```python
from build123d import *

# Parameters (mm, degrees)
SKETCH1_W                = 14
SKETCH1_H                = 99
BOSS_EXTRUDE1_DEPTH      = 40
CUT_EXTRUDE1_DEPTH       = 108.689368092
SKETCH3_W                = 6
SKETCH3_H                = 5
BOSS_EXTRUDE2_DEPTH      = 6
SKETCH4_R                = 1
CUT_EXTRUDE2_DEPTH       = 6
SKETCH5_R                = 1
CUT_EXTRUDE3_DEPTH       = 6
FILLET1_R                = 2
SKETCH6_W                = 6
SKETCH6_H                = 5
BOSS_EXTRUDE3_DEPTH      = 6
SKETCH7_R                = 1
CUT_EXTRUDE4_DEPTH       = 5
SKETCH8_R                = 1
CUT_EXTRUDE5_DEPTH       = 5
FILLET2_R                = 2
SKETCH9_W                = 11
SKETCH9_H                = 5.6
CUT_EXTRUDE6_DEPTH       = 10
BOSS_EXTRUDE4_DEPTH      = 4
BOSS_EXTRUDE4_DEPTH_BACK = 7
FILLET4_R                = 4
SKETCH11_W               = 14.2
SKETCH11_H               = 1.6
BOSS_EXTRUDE5_DEPTH      = 5
SKETCH12_W               = 2
SKETCH12_H               = 2.5
BOSS_EXTRUDE6_DEPTH      = 1
SKETCH13_W               = 2
SKETCH13_H               = 2.5
BOSS_EXTRUDE7_DEPTH      = 1
BOSS_EXTRUDE8_DEPTH      = 10
BOSS_EXTRUDE9_DEPTH      = 10


with BuildPart() as part:
    # Sketch1 → Boss-Extrude1 (new body)
    with BuildSketch(Plane(origin=(0, 0, 0), x_dir=(1, 0, 0), z_dir=(0, 1, 0))):
        with Locations((7, 49.5)):
            Rectangle(SKETCH1_W, SKETCH1_H)
    extrude(amount=BOSS_EXTRUDE1_DEPTH)

    # Sketch2 → Cut-Extrude1 (cut, through all)
    with BuildSketch(Plane.XY):
        with BuildLine():
            Line((14, 0), (14, 40))
            Line((14, 40), (2, 40))
            add(Edge.make_bspline(
                [(2, 40), (2.539521764, 17.05373231), (14, 0)],
                knots=[0, 0, 0, 0.735735095, 0.735735095, 0.735735095], degree=2))
        make_face()
    extrude(amount=-CUT_EXTRUDE1_DEPTH, mode=Mode.SUBTRACT)

    # Sketch3 → Boss-Extrude2 (add)
    with BuildSketch(Plane.ZY):
        with Locations((-84.5, 10)):
            Rectangle(SKETCH3_W, SKETCH3_H)
        with Locations((-14.5, 10)):
            Rectangle(SKETCH3_W, SKETCH3_H)
    extrude(amount=BOSS_EXTRUDE2_DEPTH)

    # Sketch4 → Cut-Extrude2 (cut)
    with BuildSketch(Plane.XZ.offset(-7.5)):
        with Locations(Location((-3, -84.5, 0), (0, 0, 270))):
            Circle(SKETCH4_R)
    extrude(amount=-CUT_EXTRUDE2_DEPTH, mode=Mode.SUBTRACT)

    # Sketch5 → Cut-Extrude3 (cut)
    with BuildSketch(Plane.XZ.offset(-7.5)):
        with Locations(Location((-3, -14.5, 0), (0, 0, 270))):
            Circle(SKETCH5_R)
    extrude(amount=-CUT_EXTRUDE3_DEPTH, mode=Mode.SUBTRACT)

    # Fillet1
    fillet1_edges = [part.edges().sort_by_distance(p)[0] for p in [
        (0, 10, -81.5),
        (0, 10, -87.5),
        (-6, 10, -81.5),
        (-6, 10, -87.5),
        (0, 10, -17.5),
        (0, 10, -11.5),
        (-6, 10, -17.5),
        (-6, 10, -11.5),
    ]]
    fillet(fillet1_edges, radius=FILLET1_R)

    # Sketch6 → Boss-Extrude3 (add)
    with BuildSketch(Plane.ZY):
        with Locations((-69.5, 27)):
            Rectangle(SKETCH6_W, SKETCH6_H)
        with Locations((-29.5, 27)):
            Rectangle(SKETCH6_W, SKETCH6_H)
    extrude(amount=BOSS_EXTRUDE3_DEPTH)

    # Sketch7 → Cut-Extrude4 (cut)
    with BuildSketch(Plane(origin=(0, 29.5, 0), x_dir=(1, 0, 0), z_dir=(0, 1, 0))):
        with Locations(Location((-3, 69.5, 0), (0, 0, 270))):
            Circle(SKETCH7_R)
    extrude(amount=-CUT_EXTRUDE4_DEPTH, mode=Mode.SUBTRACT)

    # Sketch8 → Cut-Extrude5 (cut)
    with BuildSketch(Plane(origin=(0, 29.5, 0), x_dir=(1, 0, 0), z_dir=(0, 1, 0))):
        with Locations(Location((-3, 29.5, 0), (0, 0, 270))):
            Circle(SKETCH8_R)
    extrude(amount=-CUT_EXTRUDE5_DEPTH, mode=Mode.SUBTRACT)

    # Fillet2
    fillet2_edges = [part.edges().sort_by_distance(p)[0] for p in [
        (0, 27, -66.5),
        (0, 27, -72.5),
        (-6, 27, -66.5),
        (-6, 27, -72.5),
        (0, 27, -32.5),
        (0, 27, -26.5),
        (-6, 27, -32.5),
        (-6, 27, -26.5),
    ]]
    fillet(fillet2_edges, radius=FILLET2_R)

    # Sketch9 → Cut-Extrude6 (cut)
    with BuildSketch(Plane.ZY):
        with Locations((-81.5, 26.7)):
            Rectangle(SKETCH9_W, SKETCH9_H)
        with Locations((-17.5, 26.7)):
            Rectangle(SKETCH9_W, SKETCH9_H)
    extrude(amount=-CUT_EXTRUDE6_DEPTH, mode=Mode.SUBTRACT)

    # Sketch10 → Boss-Extrude4 (add, two sides: drawn at the far end of the back side and taken through both)
    with BuildSketch(Plane.ZY.offset(-BOSS_EXTRUDE4_DEPTH_BACK)):
        Polygon((-76, 29.5), (-74.4, 29.5), (-74.4, 22.3), (-76, 22.3), (-88.6, 22.3), (-88.6, 29.5), (-87, 29.5), (-87, 23.9), (-76, 23.9), align=None)
        Polygon((-23, 29.5), (-24.6, 29.5), (-24.6, 22.3), (-23, 22.3), (-10.4, 22.3), (-10.4, 29.5), (-12, 29.5), (-12, 23.9), (-23, 23.9), align=None)
    extrude(amount=BOSS_EXTRUDE4_DEPTH + BOSS_EXTRUDE4_DEPTH_BACK)

    # Fillet4
    fillet4_edges = [part.edges().sort_by_distance(p)[0] for p in [
        (0, 22.3, -81.5),
        (0, 22.3, -17.5),
    ]]
    fillet(fillet4_edges, radius=FILLET4_R - 0.0001)  # a hair under: the kernel refuses the full size

    # Sketch11 → Boss-Extrude5 (add)
    with BuildSketch(Plane.ZY):
        with Locations((-81.5, 30.3)):
            Rectangle(SKETCH11_W, SKETCH11_H)
        with Locations((-17.5, 30.3)):
            Rectangle(SKETCH11_W, SKETCH11_H)
    extrude(amount=-BOSS_EXTRUDE5_DEPTH)

    # Sketch12 → Boss-Extrude6 (add)
    with BuildSketch(Plane.XZ.offset(-29.5)):
        with Locations((4, -77.25)):
            Rectangle(SKETCH12_W, SKETCH12_H)
        with Locations((4, -85.75)):
            Rectangle(SKETCH12_W, SKETCH12_H)
    extrude(amount=BOSS_EXTRUDE6_DEPTH)

    # Sketch13 → Boss-Extrude7 (add)
    with BuildSketch(Plane.XZ.offset(-29.5)):
        with Locations((4, -13.25)):
            Rectangle(SKETCH13_W, SKETCH13_H)
        with Locations((4, -21.75)):
            Rectangle(SKETCH13_W, SKETCH13_H)
    extrude(amount=BOSS_EXTRUDE7_DEPTH)

    # Sketch14 → Boss-Extrude8 (add)
    with BuildSketch(Plane.XZ.offset(-22.3)):
        Polygon((4.247690058, -10.4), (7, -10.4), (7, -24.6), (4.247690059, -24.6), align=None)
    extrude(amount=BOSS_EXTRUDE8_DEPTH)

    # Sketch15 → Boss-Extrude9 (add)
    with BuildSketch(Plane.XZ.offset(-22.3)):
        Polygon((4.247690058, -74.4), (4.247690059, -88.6), (7, -88.6), (7, -74.4), align=None)
    extrude(amount=BOSS_EXTRUDE9_DEPTH)


solid = part.part
```
Read the model definition and answer for the solid it produces. Units are mm, in the model's axes. A direction names the side the tool comes from. Coordinates: 2 decimals unless noted, no trailing zeros. Answer as a JSON object with one key per item and string values.
Q1. A tool of negligible diameter and unlimited length cuts with its end or side. For faces 1 (the flat face through (2, 23.9, -17)), 2 (the flat face through (-3, 7.5, -13)), 3 (the cylindrical face through (-1.203, 21.159, -81.599)), from which of +Z, -Z, +X, -X, +Y, -Y can it reach the whole face along a straight path? Write none if from no direction.
The answers:
{"face 1": "+X, -X", "face 2": "+Z, -Z, -X, -Y", "face 3": "+Z, -Z, -X"}
Q2. Flat-ended cylindrical pins translate along their axes: pin 1 Ø3 at (x, z) = (-2, -67.5) entering from -Y; pin 2 Ø5 at (x, z) = (-2, -29.5) entering from -Y; pin 3 Ø1.1 at (x, y) = (4, 29) entering from -Z; pin 4 Ø8 at (y, z) = (25, -79.5) entering from -X. Find the tip coordinate at first contact, or state that the pin passes through.
The answers:
{"pin 1": "stops at y = 24.5", "pin 2": "stops at y = 0", "pin 3": "stops at z = -88.6", "pin 4": "stops at x = -4"}
Q3. The part is cut by section A-A on y = 27. Give the number of separate pieces and of enclosed holes in the cut face, then the cut area to 3 significant figures.
The answers:
{"separate pieces": "3", "enclosed holes": "2", "area": "367 mm2"}
Q4. Determine the mould class of faces 4 (the flat face through (-6, 10, -85)), 5 (the cylindrical face through (-5.4, 10.04, -82.07)), 6 (the flat face through (2, 27, -87)) for opening direction Z: pulls with the +Z half, pulls with the -Z half, needs draft (parallel to the pull), parting line crosses it, or undercut.
The answers:
{"face 4": "needs draft", "face 5": "undercut", "face 6": "undercut"}
Q5. Consider line 1 (Z direction, x = 4.75, y = 27.5); line 2 (X direction, y = 26.1, z = -29.5); line 3 (X direction, y = 27.65, z = -69.5). Determine where each line is inside the solid, lowest interval first. Write a range as [from, to].
The answers:
{"line 1": "z = [-88.6, -87], [-76, -74.4], [-24.6, -23], [-12, -10.4]", "line 2": "x = [-6, -4], [-2, 3.43]", "line 3": "x = [-6, -4], [-2, 3.15]"}
